The listing builds one solid part. Answer for the finished solid, in the listing's coordinates (mm). A direction names the side the tool comes from. Give positions to 0.01 mm unless a question says otherwise; leave off trailing zeros. Loops run counter-clockwise (first coordinate to the right, second up) from the corner with the lowest first, then second, coordinate; pieces in that order, holes last. Notation, with made-up numbers: (22, 10.5) - (68, 10.5) arc R25 cw to (68, 33.5) - close; hole circle Ø10 at (-18, -14). An arc over 180 degrees is marked (long way). Write each question's results on one line, items separated by ' | '.
from build123d import *

# Parameters (mm, degrees)
F0_W          = 50
F0_H          = 50
F0_R          = 2.5
F1_DEPTH      = 5
F0_W_2        = 4.7625
F0_H_2        = 4.7625
F2_DEPTH      = 2.38125
F3_DEPTH      = 5
F4_DEPTH      = 15
F4_DEPTH_BACK = 5


with BuildPart() as f1:
    # F0 (on Top) → F1 (new body, symmetric)
    with BuildSketch(Plane.XY):
        with Locations((25, -25)):
            Rectangle(F0_W, F0_H)
        with Locations((5, -45)):
            Circle(F0_R, mode=Mode.SUBTRACT)
        Polygon((18.098719, -22.61875), (22.61875, -22.61875), (22.61875, -12.242739), (39.545106, -12.242739), (39.545106, -17.005239), (39.545106, -38.55984), (34.782606, -38.55984), (30.020106, -38.55984), (30.020106, -33.79734), (34.782606, -33.79734), (34.782606, -17.005239), (27.38125, -17.005239), (27.38125, -22.61875), (27.38125, -25), (27.38125, -27.38125), (25, -27.38125), (22.61875, -27.38125), (18.098719, -27.38125), (13.336219, -27.38125), (13.336219, -14.235092), (4.879977, -14.235092), (4.879977, -9.472592), (4.879977, -5.390268), (9.642477, -5.390268), (9.642477, -9.472592), (13.336219, -9.472592), (18.098719, -9.472592), (18.098719, -14.235092), align=None, mode=Mode.SUBTRACT)
        with Locations((45, -5)):
            Circle(F0_R, mode=Mode.SUBTRACT)
    extrude(amount=F1_DEPTH, both=True)

    # F0 (on Top) → F2 (cut)
    with BuildSketch(Plane.XY):
        Polygon((22.61875, -27.38125), (22.61875, -25), (22.61875, -22.61875), (18.098719, -22.61875), (18.098719, -14.235092), (18.098719, -9.472592), (13.336219, -9.472592), (9.642477, -9.472592), (9.642477, -5.390268), (4.879977, -5.390268), (4.879977, -9.472592), (4.879977, -14.235092), (13.336219, -14.235092), (13.336219, -27.38125), (18.098719, -27.38125), align=None)
        Polygon((22.61875, -12.242739), (22.61875, -22.61875), (25, -22.61875), (27.38125, -22.61875), (27.38125, -17.005239), (34.782606, -17.005239), (34.782606, -33.79734), (34.782606, -38.55984), (39.545106, -38.55984), (39.545106, -17.005239), (39.545106, -12.242739), align=None)
        with Locations((32.401356, -36.17859)):
            Rectangle(F0_W_2, F0_H_2)
    extrude(amount=F2_DEPTH, mode=Mode.SUBTRACT)

    # F0 (on Top) → F3 (join)
    with BuildSketch(Plane.XY):
        Polygon((22.61875, -12.242739), (22.61875, -22.61875), (25, -22.61875), (27.38125, -22.61875), (27.38125, -17.005239), (34.782606, -17.005239), (34.782606, -33.79734), (34.782606, -38.55984), (39.545106, -38.55984), (39.545106, -17.005239), (39.545106, -12.242739), align=None)
        with Locations((32.401356, -36.17859)):
            Rectangle(F0_W_2, F0_H_2)
        Polygon((22.61875, -27.38125), (22.61875, -25), (22.61875, -22.61875), (18.098719, -22.61875), (18.098719, -14.235092), (18.098719, -9.472592), (13.336219, -9.472592), (9.642477, -9.472592), (9.642477, -5.390268), (4.879977, -5.390268), (4.879977, -9.472592), (4.879977, -14.235092), (13.336219, -14.235092), (13.336219, -27.38125), (18.098719, -27.38125), align=None)
    extrude(amount=-F3_DEPTH)

    # F0 (on Top) → F4 (join, two sides)
    with BuildSketch(Plane.XY) as f4_sk:
        with Locations((5, -45)):
            Circle(F0_R)
        with Locations((45, -5)):
            Circle(F0_R)
    extrude(amount=F4_DEPTH)
    extrude(f4_sk.sketch, amount=-F4_DEPTH_BACK)


solid = f1.part
Item 1: Flat-ended cylindrical pins translate along their axes: P1, Ø1, axis at x = 9.5, y = -30, coming from the +Z side; P2, Ø6, axis at y = -43.5, z = 11.5, coming from the -X side; P3, Ø1, axis at x = 31.5, z = 6.5, coming from the -Y side. Find the tip coordinate at first contact, or state that the pin passes through.
Values found:
P1: stops at z = 5 | P2: stops at x = 2.5 | P3: passes through
Item 2: A cutting plane is placed at A-A, the plane z = 3.25. Determine the outline of the cut face in (x, y), plus the area to 3 significant figures.
Values found:
outline: (0, -50) - (50, -50) - (50, 0) - (0, 0) - close; hole (4.88, -14.24) - (13.34, -14.24) - (13.34, -27.38) - (27.38, -27.38) - (27.38, -17.01) - (34.78, -17.01) - (34.78, -33.8) - (30.02, -33.8) - (30.02, -38.56) - (39.55, -38.56) - (39.55, -12.24) - (22.62, -12.24) - (22.62, -22.62) - (18.1, -22.62) - (18.1, -9.47) - (9.64, -9.47) - (9.64, -5.39) - (4.88, -5.39) - close | area: 2,080 mm²
Item 3: For faces 5 (the face through (25, -50, 0)), 6 (the face through (31, -17.005, 2)), determine the directions among +Z, -Z, +X, -X, +Y, -Y from which every point of the face is accessible in a straight line to the end or side of a thin tool.
Values found:
face 5: +Z, -Z, +X, -X, -Y | face 6: +Z
Item 4: For a pull along Y with two mould halves and no side action, classify faces 1 (the face through (0, -25, 0)), 2 (the face through (4.88, -10, 3)), 3 (the face through (31, -12.243, 3)), 4 (the face through (4.46, -47.44, 9.93)) as released by +Y, released by -Y, zero draft, split by the parting line, or undercut.
Values found:
face 1: zero draft | face 2: undercut | face 3: undercut | face 4: split by the parting line
Item 5: A cutting plane is placed at D-D, the plane z = 10.25. Determine the outline of the cut face in (x, y), plus the area to 3 significant figures.
Values found:
outline: circle Ø5 at (5, -45); circle Ø5 at (45, -5) | area: 39.3 mm²
Item 6: A cutting plane is placed at B-B, the plane y = -45. Determine the outline of the cut face in (x, z), plus the area to 3 significant figures.
Values found:
outline: (0, -5) - (50, -5) - (50, 5) - (7.5, 5) - (7.5, 15) - (2.5, 15) - (2.5, 5) - (0, 5) - close | area: 550 mm²
Item 7: Find the intervals of material crossed by line 1 along X through (y, z) = (-21.5, 1.5); line 2 along Y through (x, z) = (25.5, -1.75); line 3 along X through (y, z) = (-9, 3.25), in increasing order. Write a range as [from, to].
Values found:
line 1: x = [0, 13.34], [18.1, 22.62], [27.38, 34.78], [39.55, 50] | line 2: y = [-50, -27.38], [-22.62, 0] | line 3: x = [0, 4.88], [9.64, 50]
Item 8: A cutting plane is placed at C-C, the plane x = 9. Determine the outline of the cut face in (y, z).
Values found:
outline: (-50, -5) - (0, -5) - (0, 5) - (-5.39, 5) - (-5.39, 0) - (-14.24, 0) - (-14.24, 5) - (-50, 5) - close
